Source: CAD feature listing. Evaluate the final solid. Frame: model axes, mm. Round coordinates to 2 decimals unless told otherwise and drop trailing zeros. Order: outer loops, then holes, each group sorted by start corner. A loop starts at its lowest first (then second) coordinate and runs counter-clockwise, first axis right, second up. Notation, with made-up numbers: (-29, 34.25) -> (-24, 34.25) arc R24 ccw to (-24, 68.25) -> close; hole circle Ø9 at (59.25, -35). An arc over 180 degrees is marked (long way). One line per item, written item: value. Start each with the question number.
1) Section D-D (z = 2). State how many separate pieces and enclosed holes the cut face has, and give its area (3 significant figures).
2) Section B-B (y = 132.5). Return the cut outline in (x, z).
3) Section C-C (x = 57.5). Return the cut outline in (y, z).
4) Mould query, pull axis X, two halves, no side actions, for faces 1 (the face through (-224.782, 9.893, 4.93)), 2 (the face through (160.498, -135.414, 5.07)), 3 (the face through (-3, -97, 0)). Classes: pulls with the +X half, pulls with the -X half, needs draft (parallel to the pull), parting line crosses it, or undercut.
5) Pin query (flat end, axial travel): P1, Ø5, axis at y = 124, z = 3, coming from the -X side; P2, Ø3, axis at x = 36.5, y = -100.5, coming from the -Z side; P3, Ø2, axis at x = -65.5, z = 4.5, coming from the +Y side; P4, Ø5, axis at x = -116.5, z = 7, coming from the +Y side. Return the tip coordinate at first contact, or that it passes through.
6) Ray query, L1, parallel to Y at x = 0, z = 5.25; L2, parallel to X at y = -153, z = 5.25; L3, parallel to X at y = 202.5, z = 5. Return the intervals inside material, ascending.
7) Section A-A (x = 149). Return the cut outline in (y, z), and give its area (3 significant figures).
```python
from build123d import *

# Parameters (mm, degrees)
F0_R     = 225
F1_DEPTH = 10
F2_R     = 80
F2_R_2   = 3
F2_R_3   = 20
F3_DEPTH = 10.001


with BuildPart() as f1:
    # F0 (on Top) → F1 (new body)
    with BuildSketch(Plane.XY):
        Circle(F0_R)
    extrude(amount=F1_DEPTH)

    # F2 (on face) → F3 (cut, through all)
    with BuildSketch(Plane.XY.offset(10)):
        Circle(F2_R)
        with Locations((-95, 0)):
            Circle(F2_R_2)
        with Locations((-165, 0)):
            Circle(F2_R_2)
        with Locations((0, -95)):
            Circle(F2_R_2)
        with Locations((0, -165)):
            Circle(F2_R_2)
        with Locations((0, 165)):
            Circle(F2_R_2)
        with Locations((0, 95)):
            Circle(F2_R_2)
        with Locations((95, 0)):
            Circle(F2_R_2)
        with Locations((165, 0)):
            Circle(F2_R_2)
        with Locations((-141.421356, -141.421356)):
            Circle(F2_R_3)
        with Locations((-141.421356, 141.421356)):
            Circle(F2_R_3)
        with Locations((141.421356, -141.421356)):
            Circle(F2_R_3)
        with Locations((141.421356, 141.421356)):
            Circle(F2_R_3)
    extrude(amount=-F3_DEPTH, mode=Mode.SUBTRACT)


solid = f1.part
```
Findings:
1. separate pieces: 1
1. enclosed holes: 13
1. area: 134,000 mm2
2. outline: (-181.85, 0) -> (-159.32, 0) -> (-159.32, 10) -> (-181.85, 10) -> close; (-123.52, 0) -> (123.52, 0) -> (123.52, 10) -> (-123.52, 10) -> close; (159.32, 0) -> (181.85, 0) -> (181.85, 10) -> (159.32, 10) -> close
3. outline: (-217.53, 0) -> (-55.62, 0) -> (-55.62, 10) -> (-217.53, 10) -> close; (55.62, 0) -> (217.53, 0) -> (217.53, 10) -> (55.62, 10) -> close
4. face 1: parting line crosses it
4. face 2: undercut
4. face 3: needs draft
5. P1: x = -189.37
5. P2: z = 0
5. P3: y = 215.56
5. P4: y = 193.98
6. L1: -225 to -168, -162 to -98, -92 to -80, 80 to 92, 98 to 162, 168 to 225
6. L2: -164.97 to -157.73, -125.11 to 125.11, 157.73 to 164.97
6. L3: -98.08 to 98.08
7. outline: (-168.59, 0) -> (-159.93, 0) -> (-159.93, 10) -> (-168.59, 10) -> close; (-122.91, 0) -> (122.91, 0) -> (122.91, 10) -> (-122.91, 10) -> close; (159.93, 0) -> (168.59, 0) -> (168.59, 10) -> (159.93, 10) -> close
7. area: 2,630 mm2
